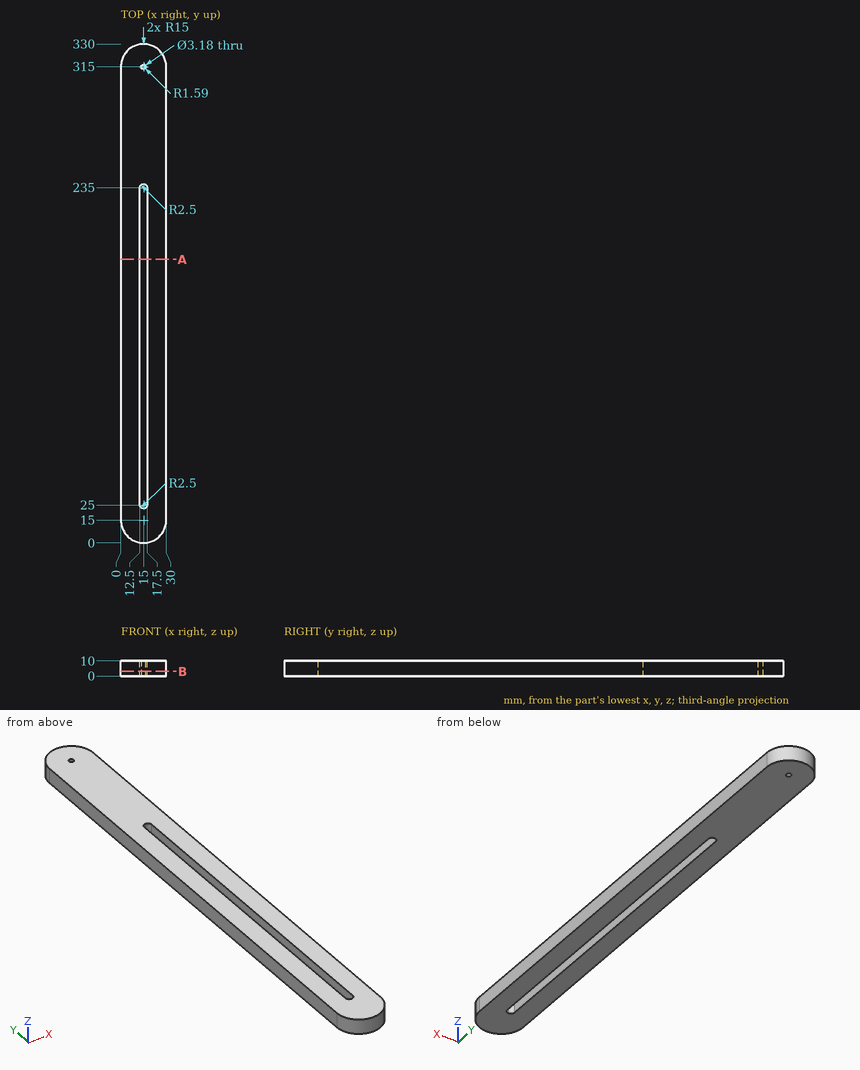
Geometry check sheet. Reference: drawing and pictorial views, mm from the part's lowest x, y, z. Coordinates: 2 decimals unless noted, no trailing zeros. Order: outer loops, then holes, each group sorted by start corner. A loop starts at its lowest first (then second) coordinate and runs counter-clockwise, first axis right, second up. Notation, with made-up numbers: (76, -14.5) -> (88, -14.5) arc R17 ccw to (88, -1.5) -> close; hole circle Ø1 at (53.25, 71). An arc over 180 degrees is marked (long way). Put each result on its own line as item: value. Start each with the question number.
1) Cross-section at A-A (y = 187.5). Enter the section's corners in (x, z), plus the area to 3 significant figures.
2) Cross-section at B-B (z = 3). Enter the section's corners in (x, y).
3) Go/stop test with flat-tipped pins: pin 1 (3 mm diameter, centred on x = 17.5, z = 9, fed in from +Y); pin 2 (3 mm diameter, centred on x = 4, z = 5.5, fed in from -Y); pin 3 (1.5 mm diameter, centred on x = 10.5, z = 6, fed in from +Y). Record where each tip stops, or that it passes through.
4) Material ranges on L1, parallel to X at y = 315, z = 4; L2, parallel to X at y = 188.5, z = 2; L3, parallel to Y at x = 11, z = 9.5, recorded low to high.
Geometry check:
1. outline: (0, 0) -> (12.5, 0) -> (12.5, 10) -> (0, 10) -> close; (17.5, 0) -> (30, 0) -> (30, 10) -> (17.5, 10) -> close
1. area: 250 mm^2
2. outline: (0, 15) arc R15 ccw to (30, 15) -> (30, 315) arc R15 ccw to (0, 315) -> close; hole (12.5, 25) arc R2.5 ccw to (17.5, 25) -> (17.5, 235) arc R2.5 ccw to (12.5, 235) -> close; hole circle Ø3.18 at (15, 315)
3. pin 1: stops at y = 329.97
3. pin 2: stops at y = 3.39
3. pin 3: stops at y = 329.52
4. L1: x = 0 to 13.41, 16.59 to 30
4. L2: x = 0 to 12.5, 17.5 to 30
4. L3: y = 0.54 to 329.46
